Can you work these out from the model? Positions are in its coordinate system, mm. A direction names the side the tool comes from. Give positions to 0.01 mm unless a question says otherwise; leave off trailing zeros. Order: outer loops, then holes, each group sorted by start corner. A loop starts at its lowest first (then second) coordinate and runs counter-clockwise, first axis right, second up. Notation, with made-up numbers: (55, -31.75) - (74, -31.75) arc R15 cw to (74, -24.75) - close; hole circle Ø1 at (-8, 53.5). An arc over 180 degrees is marked (long way). Return JSON: item names as keys, results as strings.
```python
from build123d import *

# Parameters (mm, degrees)
F0_R     = 12.065
F1_DEPTH = 3.81
F2_R     = 9.652
F3_DEPTH = 11.43
F4_R     = 12.065
F5_DEPTH = 3.81


with BuildPart() as f1:
    # F0 (on Front) → F1 (new body)
    with BuildSketch(Plane.XZ):
        Circle(F0_R)
    extrude(amount=-F1_DEPTH)

    # F2 (on face) → F3 (join)
    with BuildSketch(Plane.XZ):
        Circle(F2_R)
    extrude(amount=F3_DEPTH)

    # F4 (on face) → F5 (join)
    with BuildSketch(Plane.XZ.offset(11.43)):
        Circle(F4_R)
    extrude(amount=F5_DEPTH)


solid = f1.part
```
1. Suppose I cut it at B-B (z = 0). List the corners of the cut face in (x, y) for me (3 decimals).
Checks:
{"outline": "(-12.065, -15.24) - (12.065, -15.24) - (12.065, -11.43) - (9.652, -11.43) - (9.652, 0) - (12.065, 0) - (12.065, 3.81) - (-12.065, 3.81) - (-12.065, 0) - (-9.652, 0) - (-9.652, -11.43) - (-12.065, -11.43) - close"}
2. Suppose I cut it at D-D (y = -6). List the corners of the cut face in (x, z) for me, plus the area to 3 significant figures.
Checks:
{"outline": "circle Ø19.3 at (0, 0)", "area": "293 mm^2"}
3. On a 3-axis mill with a long thin cutter (end or side, diameter ignored), from which of +Z, -Z, +X, -X, +Y, -Y can I reach the whole of each face in a straight line? I mean faces 1 (the face through (4, -11.43, 9)), 2 (the face through (11.51, 1.88, 3.62)). Say none if no direction works.
Checks:
{"face 1": "none", "face 2": "+Y, -Y"}
4. Suppose I cut it at C-C (y = -13.75). List the corners of the cut face in (x, z) for me (3 decimals), plus the area to 3 significant figures.
Checks:
{"outline": "circle Ø24.13 at (0, 0)", "area": "457 mm^2"}
5. Thinking about a two-plate mould opening in Y: for faces 3 (the face through (11.51, -13.31, 3.62)), 4 (the face through (-7.66, -5.63, -5.87)), 5 (the face through (0, 3.81, 0)), which applies, +Y half, -Y half, draft (parallel to the pull), parting line (faces both ways), or undercut?
Checks:
{"face 3": "draft", "face 4": "undercut", "face 5": "+Y half"}
6. Suppose I cut it at A-A (x = 0). List the corners of the cut face in (y, z) for me (3 decimals).
Checks:
{"outline": "(-15.24, -12.065) - (-11.43, -12.065) - (-11.43, -9.652) - (0, -9.652) - (0, -12.065) - (3.81, -12.065) - (3.81, 12.065) - (0, 12.065) - (0, 9.652) - (-11.43, 9.652) - (-11.43, 12.065) - (-15.24, 12.065) - close"}
7. For pin 1 Ø1 at (x, y) = (-8.5, 1.5) entering from -Z; pin 2 Ø2 at (x, y) = (7, -3.5) entering from +Z, each with a flat end and sliding along its axis, tell me the tip position at first contact or that it passes through.
Checks:
{"pin 1": "z = -9.03", "pin 2": "z = 7.56"}
8. If I drill on L1, parallel to Y at x = -9.5, z = 3.75; L2, parallel to X at y = -4, z = 0.25; L3, parallel to Z at x = 2.25, y = -13.5, over which ranges is the centre line in solid material (lowest first)? Write a range as [from, to].
Checks:
{"L1": "[-15.24, -11.43], [0, 3.81]", "L2": "[-9.65, 9.65]", "L3": "[-11.85, 11.85]"}
